Source: three-view drawing plus pictorial views. Frame: mm from the lowest corner of the part. Round coordinates to 2 decimals unless told otherwise and drop trailing zeros. Order: outer loops, then holes, each group sorted by start corner. A loop starts at its lowest first (then second) coordinate and runs counter-clockwise, first axis right, second up. Notation, with made-up numbers: (26, 31.5) - (47, 31.5) arc R25 ccw to (47, 65.5) - close; hole circle Ø7 at (54, 71). An arc over 180 degrees is marked (long way). Use one line per item in the form item = value. Start each with the question number.
Q1. Ray query, line 1 (Y direction, x = 21, z = 1.15); line 2 (X direction, y = 17, z = 0.9); line 3 (X direction, y = 18.5, z = 1.55). Return the intervals inside material, ascending. Write a range as [from, to].
Q2. Cut plane B-B, the plane y = 17. Return the cut outline in (x, z).
Q3. Cut plane A-A, the plane x = 21. Return the cut outline in (y, z), and give its area (3 significant figures).
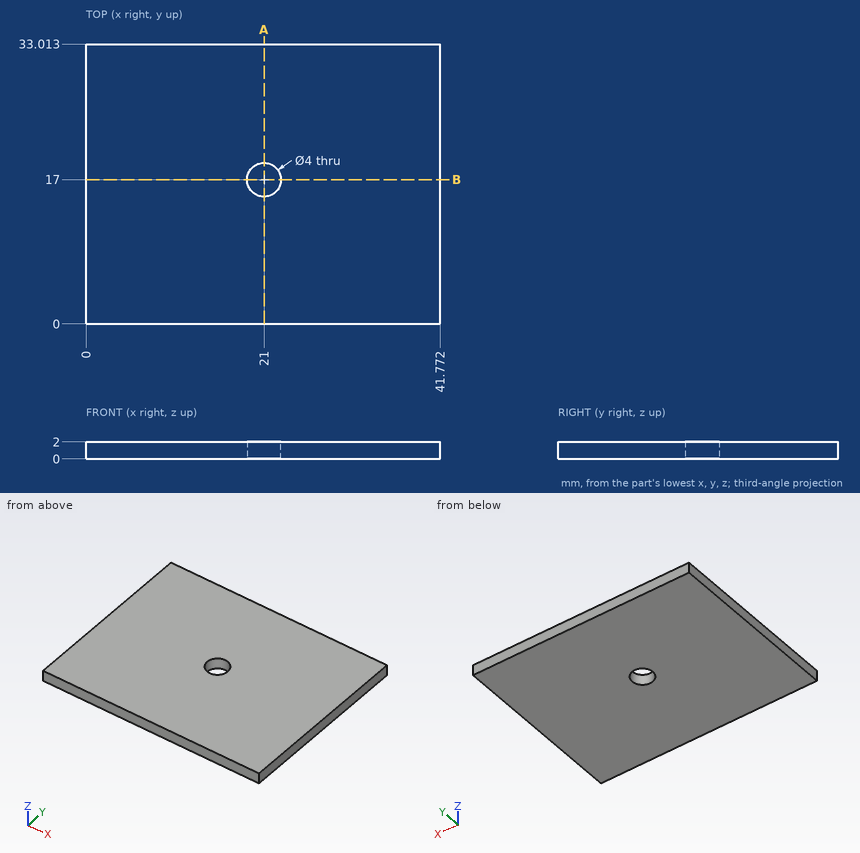
Completed:
q1.line_1 = [0, 15], [19, 33.01]
q1.line_2 = [0, 19], [23, 41.77]
q1.line_3 = [0, 19.68], [22.32, 41.77]
q2.outline = (0, 0) - (19, 0) - (19, 2) - (0, 2) - close; (23, 0) - (41.77, 0) - (41.77, 2) - (23, 2) - close
q3.outline = (0, 0) - (15, 0) - (15, 2) - (0, 2) - close; (19, 0) - (33.01, 0) - (33.01, 2) - (19, 2) - close
q3.area = 58.0 mm2
